Check sheet for the modelled part. Datum: model origin and axes. Units: mm. A direction names the side the tool comes from. Round coordinates to 2 decimals unless told otherwise and drop trailing zeros. Write each loop counter-clockwise with the first axis right and the second up, starting at its lowest first coordinate (ties: lowest second). Pieces come first, ordered by that corner, then holes.
Item 1: Section check B-B, the plane z = -63. Record the cut outline in (x, y).
Item 2: Depth check by flat-ended pin: pin 1 (1.8 mm diameter, centred on y = 4.5, z = -5, fed in from +X); pin 2 (3 mm diameter, centred on x = 85.5, z = -12.5, fed in from +Y). Enter the tip coordinate at first touch or a pass-through.
Item 3: Set-up check for faces 4 (the flat face through (117, 9, -5)), 5 (the flat face through (112, 7, -5)), 6 (the flat face through (5, 6, -10)): record each of +Z, -Z, +X, -X, +Y, -Y from which the full face is reachable in a straight line by a thin tool's end or side.
Item 4: Section check A-A, the plane x = 56.5. Record the cut outline in (y, z).
Item 5: Release check for a two-part mould opening along X. For faces 1 (the flat face through (122, 2, -44)), 2 (the flat face through (5, 6, -80)), 3 (the flat face through (112, 7, -85)) record: pulls with the +X half, pulls with the -X half, needs draft (parallel to the pull), parting line crosses it, or undercut.
Item 6: Material ranges on line 1 along Z through (x, y) = (117.75, 4.5); line 2 along Y through (x, z) = (8.25, -5); line 3 along X through (y, z) = (7.25, -83.5), recorded low to high.
from build123d import *

# Parameters (mm, degrees)
SKETCH1_W           = 122
SKETCH1_H           = 90
BOSS_EXTRUDE1_DEPTH = 3
SKETCH2_W           = 10
SKETCH2_H           = 10
BOSS_EXTRUDE2_DEPTH = 6
CUT_EXTRUDE2_REACH  = 153.872
SKETCH4_R           = 1.5
CUT_EXTRUDE3_REACH  = 153.872
SKETCH5_R           = 1.5


with BuildPart() as part:
    # Sketch1 → Boss-Extrude1 (new body)
    with BuildSketch(Plane(origin=(0, 0, 0), x_dir=(1, 0, 0), z_dir=(0, 1, 0))):
        with Locations((61, 45)):
            Rectangle(SKETCH1_W, SKETCH1_H)
    extrude(amount=BOSS_EXTRUDE1_DEPTH)

    # Sketch2 → Boss-Extrude2 (add)
    with BuildSketch(Plane(origin=(0, 3, 0), x_dir=(1, 0, 0), z_dir=(0, 1, 0))):
        Polygon((0, 0), (10, 0), (10, 5.706645394), (10, 10), (7.781127404, 10), (0, 10), align=None)
        with Locations((5, 85)):
            Rectangle(SKETCH2_W, SKETCH2_H)
        with Locations((117, 85)):
            Rectangle(SKETCH2_W, SKETCH2_H)
        with Locations((117, 5)):
            Rectangle(SKETCH2_W, SKETCH2_H)
    extrude(amount=BOSS_EXTRUDE2_DEPTH)

    # Sketch4 → Cut-Extrude2 (cut, up to next)
    with BuildSketch(Plane.ZY, mode=Mode.PRIVATE) as cut_extrude2_sk1:
        with Locations((-85, 4.5)):
            Circle(SKETCH4_R)
    cut_extrude2_tool1 = extrude(cut_extrude2_sk1.sketch, amount=-CUT_EXTRUDE2_REACH, mode=Mode.PRIVATE) & part.part
    # Sketch4 → Cut-Extrude2 (cut, up to next)
    with BuildSketch(Plane.ZY, mode=Mode.PRIVATE) as cut_extrude2_sk2:
        with Locations((-5, 4.5)):
            Circle(SKETCH4_R)
    cut_extrude2_tool2 = extrude(cut_extrude2_sk2.sketch, amount=-CUT_EXTRUDE2_REACH, mode=Mode.PRIVATE) & part.part
    add(cut_extrude2_tool1.solids().sort_by_distance((0, 4.5, -85))[0], mode=Mode.SUBTRACT)
    add(cut_extrude2_tool2.solids().sort_by_distance((0, 4.5, -5))[0], mode=Mode.SUBTRACT)

    # Sketch5 → Cut-Extrude3 (cut, up to next)
    with BuildSketch(Plane(origin=(122, 0, 0), x_dir=(0, 0, -1), z_dir=(1, 0, 0)), mode=Mode.PRIVATE) as cut_extrude3_sk1:
        with Locations(Location((85, 4.5, 0), (0, 0, 180))):
            Circle(SKETCH5_R)
    cut_extrude3_tool1 = extrude(cut_extrude3_sk1.sketch, amount=-CUT_EXTRUDE3_REACH, mode=Mode.PRIVATE) & part.part
    # Sketch5 → Cut-Extrude3 (cut, up to next)
    with BuildSketch(Plane(origin=(122, 0, 0), x_dir=(0, 0, -1), z_dir=(1, 0, 0)), mode=Mode.PRIVATE) as cut_extrude3_sk2:
        with Locations(Location((5, 4.5, 0), (0, 0, 180))):
            Circle(SKETCH5_R)
    cut_extrude3_tool2 = extrude(cut_extrude3_sk2.sketch, amount=-CUT_EXTRUDE3_REACH, mode=Mode.PRIVATE) & part.part
    add(cut_extrude3_tool1.solids().sort_by_distance((122, 4.5, -85))[0], mode=Mode.SUBTRACT)
    add(cut_extrude3_tool2.solids().sort_by_distance((122, 4.5, -5))[0], mode=Mode.SUBTRACT)


solid = part.part
Values found:
1. outline: (0, 0) - (122, 0) - (122, 3) - (0, 3) - close
2. pin 1: passes through
2. pin 2: stops at y = 3
3. face 4: +Z, -Z, +X, -X, +Y
3. face 5: +Z, -Z, +Y
3. face 6: +X, -X, +Y
4. outline: (0, -90) - (3, -90) - (3, 0) - (0, 0) - close
5. face 1: pulls with the +X half
5. face 2: needs draft
5. face 3: undercut
6. line 1: z = -90 to -86.5, -83.5 to -80, -10 to -6.5, -3.5 to 0
6. line 2: y = 0 to 3, 6 to 9
6. line 3: x = 0 to 10, 112 to 122
